```python
from build123d import *

# Parameters (mm, degrees)
SKETCH1_W            = 176
SKETCH1_H            = 10
BOSS_EXTRUDE1_DEPTH  = 10
SKETCH2_W            = 10
SKETCH2_H            = 10
BOSS_EXTRUDE2_DEPTH  = 52.5
SKETCH3_W            = 10
SKETCH3_H            = 10
BOSS_EXTRUDE3_DEPTH  = 23
SKETCH4_W            = 10
SKETCH4_H            = 10
BOSS_EXTRUDE4_DEPTH  = 120
BOSS_EXTRUDE5_DEPTH  = 10
SKETCH17_W           = 10
SKETCH17_H           = 10
BOSS_EXTRUDE6_DEPTH  = 20
CUT_REVOLVE2_ANGLE   = 180
LPATTERN1_COUNT      = 3
LPATTERN1_PITCH      = 20
SKETCH23_W           = 10
SKETCH23_H           = 10
BOSS_EXTRUDE7_DEPTH  = 20
CUT_REVOLVE3_ANGLE   = 180
LPATTERN2_COUNT      = 3
LPATTERN2_PITCH      = 20
SKETCH25_W           = 10
SKETCH25_H           = 10
BOSS_EXTRUDE8_DEPTH  = 30
SKETCH27_W           = 10
SKETCH27_H           = 10
BOSS_EXTRUDE10_DEPTH = 30
SKETCH28_W           = 76
SKETCH28_H           = 38
BOSS_EXTRUDE11_DEPTH = 5
BOSS_EXTRUDE12_DEPTH = 10
CIRPATTERN2_COUNT    = 2
SKETCH31_R           = 3.5
SKETCH31_R_2         = 2.5
BOSS_EXTRUDE13_DEPTH = 2
SKETCH32_R           = 3.5
SKETCH32_R_2         = 2.5
BOSS_EXTRUDE14_DEPTH = 2
SKETCH33_R           = 2.5
CUT_EXTRUDE1_DEPTH   = 2
SKETCH34_R           = 2.5
CUT_EXTRUDE2_DEPTH   = 2
SKETCH35_W           = 2.388589586
SKETCH35_H           = 1
CUT_EXTRUDE3_DEPTH   = 2
SKETCH37_W           = 2.280099824
SKETCH37_H           = 1
CUT_EXTRUDE4_DEPTH   = 2
CUT_REVOLVE4_ANGLE   = 180
CUT_REVOLVE5_ANGLE   = 180
CUT_REVOLVE8_ANGLE   = 180
CUT_REVOLVE9_ANGLE   = 180


with BuildPart() as part:
    # Sketch1 → Boss-Extrude1 (new body)
    with BuildSketch(Plane.XY):
        with Locations((88, 5)):
            Rectangle(SKETCH1_W, SKETCH1_H)
    extrude(amount=BOSS_EXTRUDE1_DEPTH)

    # Sketch2 → Boss-Extrude2 (add)
    with BuildSketch(Plane(origin=(0, 0, 0), x_dir=(-1, 0, 0), z_dir=(0, 0, -1))):
        with Locations((-88, 5)):
            Rectangle(SKETCH2_W, SKETCH2_H)
    extrude(amount=BOSS_EXTRUDE2_DEPTH)

    # Sketch3 → Boss-Extrude3 (add)
    with BuildSketch(Plane(origin=(0, 0, 0), x_dir=(-1, 0, 0), z_dir=(0, 0, -1))):
        with Locations((-5, 5)):
            Rectangle(SKETCH3_W, SKETCH3_H)
        with Locations((-171, 5)):
            Rectangle(SKETCH3_W, SKETCH3_H)
    extrude(amount=BOSS_EXTRUDE3_DEPTH)

    # Mirror6: part across plane


with BuildPart() as part_1:
    add(part.part)
    add(part.part.mirror(Plane.XY.offset(-52.5)))

    # Sketch4 → Boss-Extrude4 (add)
    with BuildSketch(Plane.XZ):
        with Locations((88, 5)):
            Rectangle(SKETCH4_W, SKETCH4_H)
        with Locations((88, -110)):
            Rectangle(SKETCH4_W, SKETCH4_H)
    extrude(amount=BOSS_EXTRUDE4_DEPTH)

    # Sketch13 → Boss-Extrude5 (add)
    with BuildSketch(Plane.ZY.offset(-83)):
        Polygon((-105, 0), (-82, 0), (-105, -40), align=None)
        Polygon((0, -40), (0, 0), (-23, 0), align=None)
    extrude(amount=-BOSS_EXTRUDE5_DEPTH)

    # Sketch17 → Boss-Extrude6 (add)
    with BuildSketch(Plane.ZY.offset(-83)):
        with Locations((-52.5, 5)):
            Rectangle(SKETCH17_W, SKETCH17_H)
    boss_extrude6 = extrude(amount=BOSS_EXTRUDE6_DEPTH)

    # Sketch18 → Cut-Revolve2 (revolve, cut)
    with BuildSketch(Plane.XZ):
        with BuildLine():
            Line((71, -52.5), (65, -52.5))
            ThreePointArc((65, -52.5), (68, -55.5), (71, -52.5))
        make_face()
    cut_revolve2 = revolve(axis=Axis((71, 0, -52.5), (1, 0, 0)), revolution_arc=CUT_REVOLVE2_ANGLE, mode=Mode.SUBTRACT)

    # LPattern1: Boss-Extrude6, Cut-Revolve2 ×3
    with Locations(*[(-i * LPATTERN1_PITCH, 0, 0) for i in range(1, LPATTERN1_COUNT)]):
        add(boss_extrude6)
        add(cut_revolve2, mode=Mode.SUBTRACT)

    # Sketch23 → Boss-Extrude7 (add)
    with BuildSketch(Plane(origin=(93, 0, 0), x_dir=(0, 0, -1), z_dir=(1, 0, 0))):
        with Locations((52.5, 5)):
            Rectangle(SKETCH23_W, SKETCH23_H)
    boss_extrude7 = extrude(amount=BOSS_EXTRUDE7_DEPTH)

    # Sketch24 → Cut-Revolve3 (revolve, cut)
    with BuildSketch(Plane.XZ):
        with BuildLine():
            ThreePointArc((105, -52.5), (108, -49.5), (111, -52.5))
            Line((111, -52.5), (105, -52.5))
        make_face()
    cut_revolve3 = revolve(axis=Axis((111, 0, -52.5), (-1, 0, 0)), revolution_arc=CUT_REVOLVE3_ANGLE, mode=Mode.SUBTRACT)

    # LPattern2: Boss-Extrude7, Cut-Revolve3 ×3
    with Locations(*[(i * LPATTERN2_PITCH, 0, 0) for i in range(1, LPATTERN2_COUNT)]):
        add(boss_extrude7)
        add(cut_revolve3, mode=Mode.SUBTRACT)

    # Sketch25 → Boss-Extrude8 (add)
    with BuildSketch(Plane(origin=(0, 0, -115), x_dir=(-1, 0, 0), z_dir=(0, 0, -1))):
        with Locations((-88, -115)):
            Rectangle(SKETCH25_W, SKETCH25_H)
    extrude(amount=BOSS_EXTRUDE8_DEPTH)

    # Sketch27 → Boss-Extrude10 (add)
    with BuildSketch(Plane.XY.offset(10)):
        with Locations((88, -115)):
            Rectangle(SKETCH27_W, SKETCH27_H)
    extrude(amount=BOSS_EXTRUDE10_DEPTH)

    # Sketch28 → Boss-Extrude11 (add)
    with BuildSketch(Plane(origin=(0, 0, -145), x_dir=(-1, 0, 0), z_dir=(0, 0, -1))):
        with Locations((-88, -101)):
            Rectangle(SKETCH28_W, SKETCH28_H)
    extrude(amount=-BOSS_EXTRUDE11_DEPTH)

    # Sketch30 → Boss-Extrude12 (add)
    with BuildSketch(Plane.XZ):
        Polygon((93, -105), (123, -105), (93, -82), align=None)
        Polygon((93, 0), (93, -23), (123, 0), align=None)
    boss_extrude12 = extrude(amount=-BOSS_EXTRUDE12_DEPTH)

    # CirPattern2: Boss-Extrude12 ×2 about axis
    cirpattern2_axis = Axis((88, 0, -52.5), (0, 1, 0))
    for i in range(1, CIRPATTERN2_COUNT):
        add(boss_extrude12.rotate(cirpattern2_axis, i * 360 / CIRPATTERN2_COUNT))

    # Sketch31 → Boss-Extrude13 (add)
    with BuildSketch(Plane(origin=(0, 0, -115), x_dir=(-1, 0, 0), z_dir=(0, 0, -1))):
        with Locations((-88, -60)):
            Circle(SKETCH31_R)
        with Locations((-88, -60)):
            Circle(SKETCH31_R_2, mode=Mode.SUBTRACT)
    extrude(amount=BOSS_EXTRUDE13_DEPTH)

    # Sketch32 → Boss-Extrude14 (add)
    with BuildSketch(Plane.XY.offset(10)):
        with Locations((88, -60)):
            Circle(SKETCH32_R)
        with Locations((88, -60)):
            Circle(SKETCH32_R_2, mode=Mode.SUBTRACT)
    extrude(amount=BOSS_EXTRUDE14_DEPTH)

    # Sketch33 → Cut-Extrude1 (cut)
    with BuildSketch(Plane.XY.offset(-105)):
        with Locations((88, -60)):
            Circle(SKETCH33_R)
    extrude(amount=-CUT_EXTRUDE1_DEPTH, mode=Mode.SUBTRACT)

    # Sketch34 → Cut-Extrude2 (cut)
    with BuildSketch(Plane(origin=(0, 0, 0), x_dir=(-1, 0, 0), z_dir=(0, 0, -1))):
        with Locations((-88, -60)):
            Circle(SKETCH34_R)
    extrude(amount=-CUT_EXTRUDE2_DEPTH, mode=Mode.SUBTRACT)

    # Sketch35 → Cut-Extrude3 (cut)
    with BuildSketch(Plane.XY.offset(12)):
        with Locations((85.5, -60)):
            Rectangle(SKETCH35_W, SKETCH35_H)
    extrude(amount=-CUT_EXTRUDE3_DEPTH, mode=Mode.SUBTRACT)

    # Sketch37 → Cut-Extrude4 (cut)
    with BuildSketch(Plane(origin=(0, 0, -117), x_dir=(-1, 0, 0), z_dir=(0, 0, -1))):
        with Locations((-91, -60)):
            Rectangle(SKETCH37_W, SKETCH37_H)
    extrude(amount=-CUT_EXTRUDE4_DEPTH, mode=Mode.SUBTRACT)

    # Sketch40 → Cut-Revolve4 (revolve, cut)
    with BuildSketch(Plane.XZ):
        with BuildLine():
            ThreePointArc((100.558437384, -100.017733807), (103.558437384, -97.017733807), (106.558437384, -100.017733807))
            Line((106.558437384, -100.017733807), (103.558437384, -100.017733807))
            Line((103.558437384, -100.017733807), (100.558437384, -100.017733807))
        make_face()
    revolve(axis=Axis((103.558437384, 0, -100.017733807), (-1, 0, 0)), revolution_arc=CUT_REVOLVE4_ANGLE, mode=Mode.SUBTRACT)

    # Sketch20 → Cut-Revolve5 (revolve, cut)
    with BuildSketch(Plane.XZ):
        with BuildLine():
            ThreePointArc((2.994783484, -15.417059662), (5.994783484, -12.417059662), (8.994783484, -15.417059662))
            Line((8.994783484, -15.417059662), (2.994783484, -15.417059662))
        make_face()
    revolve(axis=Axis((2.994783484, 0, -15.417059662), (-1, 0, 0)), revolution_arc=CUT_REVOLVE5_ANGLE, mode=Mode.SUBTRACT)

    # Sketch42 → Cut-Revolve8 (revolve, cut)
    with BuildSketch(Plane.XZ.offset(120)):
        with BuildLine():
            Line((88, 38), (88, 32))
            ThreePointArc((88, 32), (85, 35), (88, 38))
        make_face()
    revolve(axis=Axis((88, -120, 38), (0, 0, -1)), revolution_arc=CUT_REVOLVE8_ANGLE, mode=Mode.SUBTRACT)

    # Sketch44 → Cut-Revolve9 (revolve, cut)
    with BuildSketch(Plane.XZ.offset(120)):
        with BuildLine():
            Line((88, -107), (88, -113))
            ThreePointArc((88, -113), (85, -110), (88, -107))
        make_face()
    revolve(axis=Axis((88, -120, -107), (0, 0, -1)), revolution_arc=CUT_REVOLVE9_ANGLE, mode=Mode.SUBTRACT)


solid = part_1.part
```
Input: part model. Units: mm. Frame: model coordinates. A direction names the side the tool comes from. Round coordinates to 2 decimals unless told otherwise and drop trailing zeros. Loops run counter-clockwise (first coordinate to the right, second up) from the corner with the lowest first, then second, coordinate; pieces in that order, holes last. Notation, with made-up numbers: (2.5, 70.25) -> (44.5, 70.25) arc R23 ccw to (44.5, 103.25) -> close; hole circle Ø10 at (23, 67). An arc over 180 degrees is marked (long way). Write each question's results on one line, items separated by ' | '.
1. First-contact query: P1, Ø3, axis at x = 89, z = -122, coming from the +Y side; P2, Ø5.5, axis at x = 88.5, y = -60, coming from the +Z side; P3, Ø2, axis at x = 72, z = -48.5, coming from the -Y side; P4, Ø8, axis at x = 75.5, y = -18.5, coming from the -Z side. Flat tips, straight axial feed; report the tip coordinate or a pass-through.
Geometry results:
P1: y = -110 | P2: z = 12 | P3: y = 0 | P4: through
2. Section C-C (z = -89). Return loops of the section in (x, y), and give its area (3 significant figures).
Geometry results:
outline: (0, 0) -> (10, 0) -> (10, 10) -> (0, 10) -> close; (73.87, 0) -> (83, 0) -> (83, -12.17) -> (93, -12.17) -> (93, 0) -> (102.13, 0) -> (102.13, 10) -> (73.87, 10) -> close; (166, 0) -> (176, 0) -> (176, 10) -> (166, 10) -> close | area: 604 mm2
3. Section D-D (y = -25). Return loops of the section in (x, z) (3 decimals).
Geometry results:
outline: (83, -115) -> (93, -115) -> (93, -96.375) -> (83, -96.375) -> close; (83, -8.625) -> (93, -8.625) -> (93, 10) -> (83, 10) -> close
4. Section A-A (y = -53). Return loops of the section in (x, z), and give its area (3 significant figures).
Geometry results:
outline: (83, -115) -> (93, -115) -> (93, -105) -> (83, -105) -> close; (83, 0) -> (93, 0) -> (93, 10) -> (83, 10) -> close | area: 200 mm2
5. Section B-B (y = -96.5). Return loops of the section in (x, z).
Geometry results:
outline: (50, -145) -> (126, -145) -> (126, -140) -> (50, -140) -> close; (83, -115) -> (93, -115) -> (93, -105) -> (83, -105) -> close; (83, 0) -> (93, 0) -> (93, 10) -> (83, 10) -> close
6. Ray query, line 1 (Y direction, x = 88, z = -116); line 2 (Y direction, x = 81, z = -95); line 3 (X direction, y = -60, z = 11). Return the intervals inside material, ascending. Write a range as from..to.
Geometry results:
line 1: -120..-110, -63.5..-62.5, -57.5..-56.5 | line 2: 0..10 | line 3: 90.5..91.5
7. Set-up query: faces 1 (the face through (88, -79, 0)), 2 (the face through (123, 5, -57.5)), 3 (the face through (83, 5, -35)), 4 (the face through (10, 5, -94)). Return all of +Z, -Z, +X, -X, +Y, -Y with unobstructed straight access to the full face (end or side cutting, diameter ignored); none if empty.
Geometry results:
face 1: +X, -X, -Y | face 2: +X, +Y, -Y | face 3: -X, +Y, -Y | face 4: +Y, -Y
8. Mould query, pull axis Y, two halves, no side actions, for faces 5 (the face through (88, -14, -115)), 6 (the face through (88, 0, -52)), 7 (the face through (89.84, -58.31, 0.99)), 8 (the face through (10, 5, -11)). Classes: +Y half, -Y half, draft (parallel to the pull), parting line (faces both ways), or undercut.
Geometry results:
face 5: undercut | face 6: -Y half | face 7: undercut | face 8: draft
